For this review, use the dimensioned drawing (mm, ordinates from the lowest corner) and the shaded views. A direction names the side the tool comes from. Give positions to 0.01 mm unless a question says otherwise; leave off trailing zeros. Order: outer loops, then holes, each group sorted by start corner. A loop starts at its lowest first (then second) coordinate and runs counter-clockwise, first axis right, second up. Notation, with made-up numbers: (30.5, -14.75) - (62.5, -14.75) arc R21 cw to (62.5, 10.25) - close; hole circle Ø8 at (37, 75). An arc over 180 degrees is marked (long way). Use a Markdown table: item, result. Add a question column.
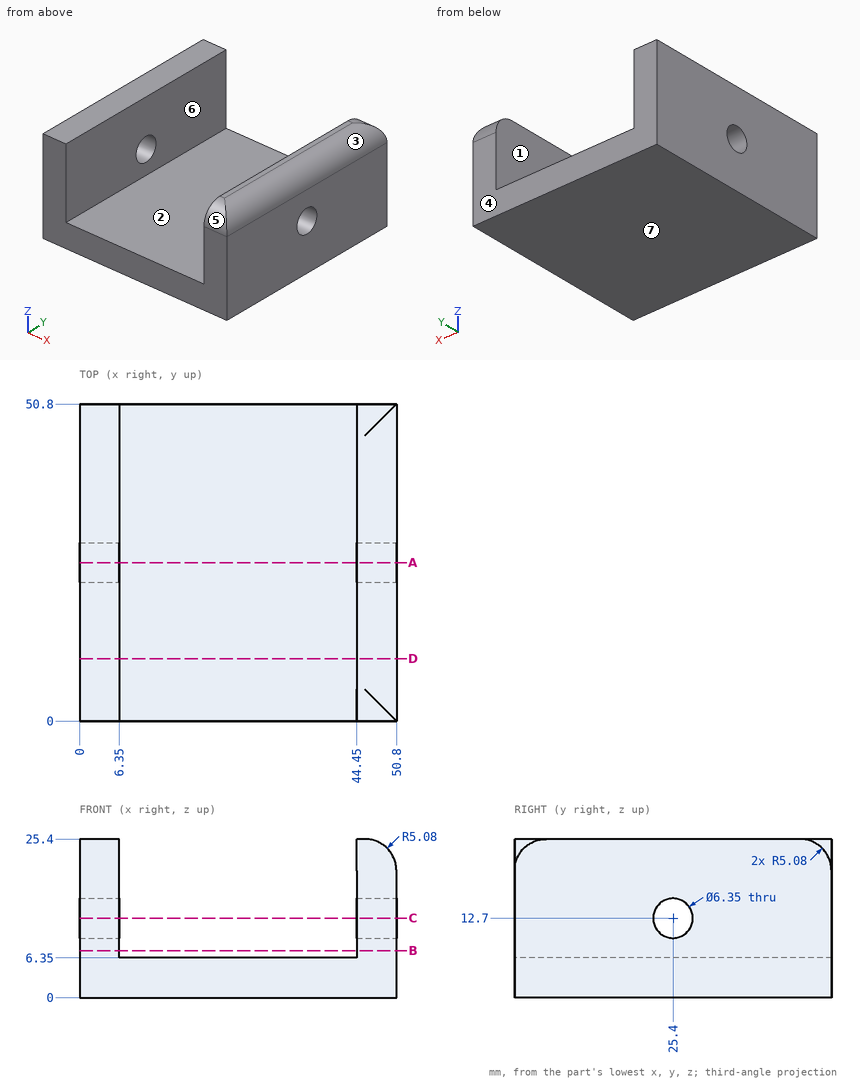
Q1. We need section D-D (y = 10). Write out the cut boundary in (x, z), plus the area to 3 significant figures.
Q2. We need section A-A (y = 25.4). Write out the cut boundary in (x, z) (3 decimals).
Q3. Draft analysis for pull direction X (two halves, no side actions). For the marked faces 1, 2, 3 and 4, state which applies: pulls with the +X half, pulls with the -X half, needs draft (parallel to the pull), parting line crosses it, or undercut.
Q4. We need section C-C (z = 12.7). Write out the cut boundary in (x, y) (3 decimals).
Q5. Clearance check with flat-ended pins moving along their axes: P1, Ø5, axis at y = 25.4, z = 12.7, coming from the -X side; P2, Ø19, axis at x = 28.5, y = 17, coming from the +Z side. State where each tip first meets the part, or that it passes through.
Q6. We need section B-B (z = 7.5). Write out the cut boundary in (x, y), plus the area to 3 significant figures.
Q7. Wall thickness on probe 1 along X at (y, z) = (26, 20.5); probe 2 along Z at (x, y) = (4.5, 25.4) (3 decimals); probe 3 along Z at (x, y) = (15.5, 18): over which ranges is each line inside the solid? List them lowest first.
Q8. Machinability: for the marked faces 5, 6 and 7, which of the approach directions +Z, -Z, +X, -X, +Y, -Y give a long, thin tool a straight path to every point of the face, cutting with its end or side? Answer none if there is none.
Here are the results:
| question | item | result |
|---|---|---|
| 1 | outline | (0, 0) - (50.8, 0) - (50.8, 20.32) arc R5.08 ccw to (45.72, 25.4) - (44.45, 25.4) - (44.45, 6.35) - (6.35, 6.35) - (6.35, 25.4) - (0, 25.4) - close |
| 1 | area | 559 mm2 |
| 2 | outline | (0, 0) - (50.8, 0) - (50.8, 9.525) - (44.45, 9.525) - (44.45, 6.35) - (6.35, 6.35) - (6.35, 9.525) - (0, 9.525) - close; (0, 15.875) - (6.35, 15.875) - (6.35, 25.4) - (0, 25.4) - close; (44.45, 15.875) - (50.8, 15.875) - (50.8, 20.32) arc R5.08 ccw to (45.72, 25.4) - (44.45, 25.4) - close |
| 3 | face 1 | undercut |
| 3 | face 2 | undercut |
| 3 | face 3 | pulls with the +X half |
| 3 | face 4 | needs draft |
| 4 | outline | (0, 0) - (6.35, 0) - (6.35, 22.225) - (0, 22.225) - close; (0, 28.575) - (6.35, 28.575) - (6.35, 50.8) - (0, 50.8) - close; (44.45, 0) - (50.8, 0) - (50.8, 22.225) - (44.45, 22.225) - close; (44.45, 28.575) - (50.8, 28.575) - (50.8, 50.8) - (44.45, 50.8) - close |
| 5 | P1 | through |
| 5 | P2 | z = 6.35 |
| 6 | outline | (0, 0) - (6.35, 0) - (6.35, 50.8) - (0, 50.8) - close; (44.45, 0) - (50.8, 0) - (50.8, 50.8) - (44.45, 50.8) - close |
| 6 | area | 645 mm2 |
| 7 | probe 1 | 0 to 6.35, 44.45 to 50.8 |
| 7 | probe 2 | 0 to 9.525, 15.875 to 25.4 |
| 7 | probe 3 | 0 to 6.35 |
| 8 | face 5 | +Z, +X, -Y |
| 8 | face 6 | +Z, +Y, -Y |
| 8 | face 7 | -Z, +X, -X, +Y, -Y |
